Model file for the job. Use its own axes, mm. A direction names the side the tool comes from. Coordinates: 2 decimals unless noted, no trailing zeros. Order: outer loops, then holes, each group sorted by start corner. A loop starts at its lowest first (then second) coordinate and runs counter-clockwise, first axis right, second up. Notation, with made-up numbers: (8, 0) - (66, 0) arc R27 ccw to (66, 24) - close; hole circle Ø1 at (87, 35.25). An arc over 180 degrees is marked (long way). Put each result on its own line as item: value. Start each with the question number.
```python
from build123d import *

# Parameters (mm, degrees)
SKETCH2_R           = 5.15
BOSS_EXTRUDE1_DEPTH = 15
SKETCH3_R           = 11
CUT_EXTRUDE1_DEPTH  = 4
SKETCH4_R           = 2.5
CUT_EXTRUDE2_DEPTH  = 9.165533085


with BuildPart() as part:
    # Sketch2 → Boss-Extrude1 (new body)
    with BuildSketch(Plane.XY):
        with BuildLine():
            Line((-16, 0), (-18, -8.234466915))
            Line((-18, -8.234466915), (-30, -8.234466915))
            Line((-30, -8.234466915), (-30, -16.4))
            Line((-30, -16.4), (30, -16.4))
            Line((30, -16.4), (30, -8.234466915))
            Line((30, -8.234466915), (18, -8.234466915))
            Line((18, -8.234466915), (16, 0))
            ThreePointArc((16, 0), (0, 16), (-16, 0))
        make_face()
        Circle(SKETCH2_R, mode=Mode.SUBTRACT)
    extrude(amount=BOSS_EXTRUDE1_DEPTH)

    # Sketch3 → Cut-Extrude1 (cut)
    with BuildSketch(Plane.XY):
        Circle(SKETCH3_R)
    extrude(amount=CUT_EXTRUDE1_DEPTH, mode=Mode.SUBTRACT)

    # Sketch4 → Cut-Extrude2 (cut, through all)
    with BuildSketch(Plane(origin=(0, -8.234466915, 0), x_dir=(1, 0, 0), z_dir=(0, 1, 0))):
        with Locations((-23, -7.5)):
            Circle(SKETCH4_R)
        with Locations((23, -7.5)):
            Circle(SKETCH4_R)
    extrude(amount=-CUT_EXTRUDE2_DEPTH, mode=Mode.SUBTRACT)


solid = part.part
```
Item 1: Wall check: line 1 along X through (y, z) = (-11.5, 7.5); line 2 along Z through (x, y) = (23, -13); line 3 along Y through (x, z) = (0, 8.5). Give the ranges that are in metal, low to high.
Item 2: Slice it at C-C, the plane y = -4. Give the cut face in (x, z).
Item 3: Pull direction Y, two halves, no side cores. Call faces 1 (the face through (4.91, 1.55, 9.42)), 2 (the face through (17.014, -4.175, 7.395)), 3 (the face through (30, -12, 7)): pulls with the +Y half, pulls with the -Y half, needs draft (parallel to the pull), parting line crosses it, or undercut.
Item 4: Slice it at D-D, the plane x = 23. Give the cut face in (y, z), plus the area to 3 significant figures.
Item 5: Slice it at A-A, the plane x = 0. Give the cut face in (y, z).
Item 6: Slice it at B-B, the plane z = 2.75. Give the cut face in (x, y).
Item 7: Flat gauge pins, fed straight in: pin 1 Ø3 at (y, z) = (0.5, 12) entering from -X; pin 2 Ø1 at (y, z) = (-1, 7.5) entering from +X; pin 3 Ø2 at (y, z) = (-7, 9) entering from -X. Where does each tip first touch, or does it go through?
Item 8: 3-axis set-ups, long thin cutter, end or side, ignore diameter. For faces 4 (the face through (-25.2, -8.234, 9.1)), 5 (the face through (-30, -12, 7)), 6 (the face through (-25, -12, 9)), 7 (the face through (-2.38, -10.74, 1.97)), 8 (the face through (25.4, -8.234, 9.1)): which of +Z, -Z, +X, -X, +Y, -Y reach the whole face in a straight line?
Here are the results:
1. line 1: x = -30 to -25.5, -20.5 to 20.5, 25.5 to 30
1. line 2: z = 0 to 5, 10 to 15
1. line 3: y = -16.4 to -5.15, 5.15 to 16
2. outline: (-16.97, 0) - (-10.25, 0) - (-10.25, 4) - (-3.24, 4) - (-3.24, 15) - (-16.97, 15) - close; (3.24, 4) - (10.25, 4) - (10.25, 0) - (16.97, 0) - (16.97, 15) - (3.24, 15) - close
3. face 1: undercut
3. face 2: pulls with the +Y half
3. face 3: needs draft
4. outline: (-16.4, 0) - (-8.23, 0) - (-8.23, 5) - (-16.4, 5) - close; (-16.4, 10) - (-8.23, 10) - (-8.23, 15) - (-16.4, 15) - close
4. area: 81.7 mm^2
5. outline: (-16.4, 0) - (-11, 0) - (-11, 4) - (-5.15, 4) - (-5.15, 15) - (-16.4, 15) - close; (5.15, 4) - (11, 4) - (11, 0) - (16, 0) - (16, 15) - (5.15, 15) - close
6. outline: (-30, -16.4) - (30, -16.4) - (30, -8.23) - (18, -8.23) - (16, 0) arc R16 ccw to (-16, 0) - (-18, -8.23) - (-30, -8.23) - close; hole circle Ø22 at (0, 0)
7. pin 1: stops at x = -16.24
7. pin 2: stops at x = 16.36
7. pin 3: stops at x = -17.94
8. face 4: +Z, -Z, -X, +Y
8. face 5: +Z, -Z, -X, +Y, -Y
8. face 6: +Y, -Y
8. face 7: -Z
8. face 8: +Z, -Z, +X, +Y
